Autodesk Inventor part; units mm, degrees
ref_plane "Work Plane1" through (0, 38.1, 0) normal (0, 1, 0) x (-1, 0, 0)
ref_plane "YZ Plane" through (0, 0, 0) normal (1, 0, 0) x (0, 1, 0)
ref_plane "XY Plane" through (0, 0, 0) normal (0, 0, 1) x (1, 0, 0)
sketch "Sketch1" plane through (0, 0, 0) normal (0, 0, 1) x (1, 0, 0)
  line L0 (0, 0) -> (25.4, 0)
  line L1 (25.4, 0) -> (25.4, 76.2)
  line L2 (25.4, 76.2) -> (0, 76.2)
  line L3 (0, 76.2) -> (0, 0)
  dimension "d0" = 76.2
  dimension "d1" = 25.4
extrude "Extrusion1" add sketch "Sketch1" along normal blind 6.35
sketch "Sketch2" plane through (0, 0, 6.35) normal (0, 0, 1) x (1, 0, 0)
  line L0 (25.4, 76.2) -> (0, 76.2)
  line L1 (25.4, 0) -> (25.4, 76.2)
  line L2 (0, 76.2) -> (25.4, 76.2)
  line L3 (25.4, 76.2) -> (25.4, 53.975)
  line L4 (25.4, 53.975) -> (0, 53.975)
  line L5 (0, 53.975) -> (0, 76.2)
  line L6 (0, 0) -> (25.4, 0)
  dimension "d4" = 22.225
extrude "Extrusion2" add sketch "Sketch2" along normal blind 3.175
ref_plane "Work Plane1" through (0, 38.1, 0) normal (0, 1, 0) x (-1, 0, 0)
mirror "Mirror1" about plane through (0, 38.1, 0) normal (0, 1, 0) of "Extrusion2"
sketch "Sketch6" plane through (0, 0, 0) normal (0, 0, 1) x (1, 0, 0)
  line L0 (25.4, 76.2) -> (0, 76.2)
  line L1 (25.4, 53.975) -> (25.4, 76.2)
  line L2 (25.4, 0) -> (0, 0)
  line L3 (0, 22.225) -> (25.4, 22.225)
  line L4 (25.4, 22.225) -> (25.4, 0)
  point P0 (12.7, 9.525)
  dimension "d28" = 12.7
  dimension "d29" = 12.7
sketch "Sketch7" plane through (0, 0, 6.35) normal (0, 0, 1) x (1, 0, 0)
  line L0 (0, 53.975) -> (25.4, 53.975)
  line L1 (0, 53.975) -> (0, 22.225)
  line L2 (25.4, 0) -> (25.4, 76.2)
  point P0 (0, 0)
  point P1 (12.7, 38.1)
  point P2 (25.4, 38.1)
  dimension "d38" = 12.7
hole "Hole3" at (12.7, 38.1, 6.35) direction (0, 0, -1) diameter 6.7564 end through all countersink diameter 12.8778 countersink angle 82
hole "Hole4" at (12.7, 9.525, 0) direction (0, 0, 1) diameter 6.3754 end through all countersink diameter 12.8778 countersink angle 82
sketch "Sketch8" plane through (0, 0, 0) normal (0, 0, -1) x (-1, 0, 0)
  line L0 (-12.7, 68.2625) -> (-12.7, 65.0875) construction
  line L1 (-15.8877, 68.2625) -> (-15.8877, 65.0875)
  line L2 (-9.5123, 65.0875) -> (-9.5123, 68.2625)
  arc A0 (-9.5123, 68.2625) -> (-15.8877, 68.2625) centre (-12.7, 68.2625) ccw
  arc A1 (-15.8877, 65.0875) -> (-9.5123, 65.0875) centre (-12.7, 65.0875) ccw
  circle A2 centre (-12.7, 9.525) radius 6.4389
  point P0 (-12.7, 66.675)
  point P1 (-12.7, 66.675)
  dimension "d54" = 3.175
  dimension "d67" = 57.15
  dimension "d68" = 6.3754
extrude "Extrusion3" cut sketch "Sketch8" against normal through all contours A0 L2 A1 L1
sketch "Sketch10" plane through (0, 76.2, 0) normal (0, 1, 0) x (1, 0, 0)
  line L0 (0, 0) -> (0, -9.525)
  line L1 (25.4, 0) -> (0, 0)
  point P0 (12.7, -4.7625)
  point P1 (0, -4.7625)
  point P2 (12.7, 0)
hole "Hole5" at (12.7, 76.2, 4.7625) direction (0, -1, 0) diameter 3.9624 depth 9.525 tip angle 118
properties part number "RollerBracket" material "Aluminum 6061"
Design review of the part built by this model. Coordinates are the model's own, in mm. A direction names the side the tool comes from. Round coordinates to 2 decimals unless told otherwise and drop trailing zeros. Order: outer loops, then holes, each group sorted by start corner. A loop starts at its lowest first (then second) coordinate and runs counter-clockwise, first axis right, second up. Notation, with made-up numbers: M 24,-10 L 38,-10 A18 ccw 38,8 Z; hole C 53,22 d3. An arc over 180 degrees is marked long. Answer as CSV lines item,"result". Start each with the question number.
1) Add section B-B (y = 38.1). Give the boundary of the cut face in (x, z), then the cut area to 3 significant figures.
2) Tool access review of faces 1 (the face through (7, 42, 6.35)), 2 (the face through (12.1, 73.44, 6.65)), 3 (the face through (10.6, 70.66, 4.7)), 4 (the face through (18, 39, 0)): name each direction out of +Z, -Z, +X, -X, +Y, -Y from which nothing blocks a thin tool from reaching the whole face with its end or side.
3) Wall thickness on line 1 along X through (y, z) = (37, 1.5); line 2 along X through (y, z) = (38.1, 1.1); line 3 along Y through (x, z) = (12.7, 5.1): over which ranges is each line inside the solid? List them lowest first. Write a range as [from, to].
4) The part is to be moulded in two halves that separate along Y. For faces 5 (the face through (13, 0, 5)), 6 (the face through (13, 53.975, 8)), 7 (the face through (25.4, 38, 5)), say which applies: +Y half, -Y half, draft (parallel to the pull), parting line (faces both ways), or undercut.
5) Add section A-A (x = 12.7). Give the boundary of the cut face in (y, z) (3 decimals), then the cut area to 3 significant figures.
6) For pin 1 Ø9 at (x, y) = (12.7, 38.1) entering from +Z, flat-tipped, find the tip position at first contact; note if it passes through.
Resolved:
1,outline,"M 0,0 L 9.32,0 L 9.32,2.83 L 6.26,6.35 L 0,6.35 Z; M 16.08,0 L 25.4,0 L 25.4,6.35 L 19.14,6.35 L 16.08,2.83 Z"
1,area,"108 mm^2"
2,face 1,"+Z, +X, -X"
2,face 2,"+Y"
2,face 3,"+Z, -Z"
2,face 4,"-Z, +X, -X, +Y, -Y"
3,line 1,"[0, 9.51], [15.89, 25.4]"
3,line 2,"[0, 9.32], [16.08, 25.4]"
3,line 3,"[0, 6.34], [12.71, 32.75], [43.45, 61.9]"
4,face 5,"-Y half"
4,face 6,"undercut"
4,face 7,"draft"
5,outline,"M 0,0 L 3.086,0 L 6.337,3.74 L 6.337,9.525 L 0,9.525 Z; M 12.713,3.74 L 15.964,0 L 34.722,0 L 34.722,2.829 L 31.661,6.35 L 22.225,6.35 L 22.225,9.525 L 12.713,9.525 Z; M 41.478,0 L 61.9,0 L 61.9,9.525 L 53.975,9.525 L 53.975,6.35 L 44.539,6.35 L 41.478,2.829 Z; M 71.45,0 L 76.2,0 L 76.2,2.781 L 71.45,2.781 Z; M 71.45,6.744 L 76.2,6.744 L 76.2,9.525 L 71.45,9.525 Z"
5,area,"389 mm^2"
6,pin 1,"z = 4.12"
